```python
from build123d import *

# Parameters (mm, degrees)
SKETCH3_W          = 5
SKETCH3_H          = 2.5
CUT_EXTRUDE1_DEPTH = 14.999635526


with BuildPart() as part:
    # Sketch1 → Revolve1 (revolve)
    with BuildSketch(Plane.XY):
        with BuildLine():
            Line((5, -4.898979486), (5, -9.898979486))
            Line((5, -9.898979486), (0, -9.898979486))
            Line((0, -9.898979486), (0, -5))
            ThreePointArc((0, -5), (4.225771274, -2.672612419), (4.517539515, 2.142857143))
            Line((4.517539515, 2.142857143), (6.32455532, 3))
            ThreePointArc((6.32455532, 3), (6.903611919, -1.157645227), (5, -4.898979486))
        make_face()
    revolve1 = revolve(axis=Axis((0, 12.862963673, 0), (0, -1, 0)))

    # Sketch3 → Cut-Extrude1 (cut, symmetric)
    with BuildSketch(Plane.XY):
        with Locations((0, -8.648979486)):
            Rectangle(SKETCH3_W, SKETCH3_H)
    cut_extrude1 = extrude(amount=CUT_EXTRUDE1_DEPTH, both=True, mode=Mode.SUBTRACT)

    # Mirror1: Revolve1, Cut-Extrude1 across plane
    add(revolve1.mirror(Plane(origin=(5, -9.898979486, 0), x_dir=(0, 0, 1), z_dir=(0, 1, 0))))
    add(cut_extrude1.mirror(Plane(origin=(5, -9.898979486, 0), x_dir=(0, 0, 1), z_dir=(0, 1, 0))), mode=Mode.SUBTRACT)


solid = part.part
```
Source: CAD feature listing. Evaluate the final solid. Frame: model axes, mm. Give positions to 0.01 mm unless a question says otherwise; leave off trailing zeros. Write each loop counter-clockwise with the first axis right and the second up, starting at its lowest first coordinate (ties: lowest second). Pieces come first, ordered by that corner, then holes.
1. Material intervals for line 1 along X through (y, z) = (-11.5, 2.5); line 2 along Y through (x, z) = (4.5, -2.5); line 3 along X through (y, z) = (-3, 1.75), sorted ascending.
2. First-contact query: pin 1 (0.8 mm diameter, centred on y = -8.5, z = 0, fed in from +X); pin 2 (6 mm diameter, centred on y = -13, z = 4.5, fed in from -X); pin 3 (1 mm diameter, centred on x = -1.5, y = 0.5, fed in from +Z). Flat tips, straight axial feed; report the tip coordinate or a pass-through.
3. Section query A-A (z = 0). Return the cut outline in (x, y), then the cut area to 3 significant figures.
4. Section query C-C (y = -11.75). Return the cut outline in (x, z), then the cut area to 3 significant figures.
5. Section query D-D (y = -18.5). Return the cut outline in (x, z).
6. Section query B-B (x = 0). Return the cut outline in (y, z).
Output values:
1. line 1: x = -4.33 to -2.5, 2.5 to 4.33
1. line 2: y = -22.24 to -15.05, -4.74 to 2.44
1. line 3: x = -6.08 to -3.6, 3.6 to 6.08
2. pin 1: stops at x = 5
2. pin 2: stops at x = -4.77
2. pin 3: stops at z = 6.92
3. outline: (-6.32, -22.8) - (-4.52, -21.94) arc R5 cw (long way) to (4.52, -21.94) - (6.32, -22.8) arc R7 ccw to (5, -14.9) - (5, -4.9) arc R7 ccw to (6.32, 3) - (4.52, 2.14) arc R5 cw (long way) to (-4.52, 2.14) - (-6.32, 3) arc R7 ccw to (-5, -4.9) - (-5, -14.9) arc R7 ccw to start; hole (-2.5, -12.4) - (2.5, -12.4) - (2.5, -7.4) - (-2.5, -7.4) - close
3. area: 143 mm2
4. outline: (-2.5, -4.33) - (-2.5, 4.33) arc R5 ccw to start; (2.5, -4.33) arc R5 ccw to (2.5, 4.33) - close
4. area: 30.7 mm2
5. outline: circle Ø13.76 at (0, 0); hole circle Ø9.66 at (0, 0)
6. outline: (-22.8, -6.32) arc R7 ccw to (-14.9, -5) - (-12.4, -5) - (-12.4, 5) - (-14.9, 5) arc R7 ccw to (-22.8, 6.32) - (-21.94, 4.52) arc R5 cw (long way) to (-21.94, -4.52) - close; (-7.4, -5) - (-4.9, -5) arc R7 ccw to (3, -6.32) - (2.14, -4.52) arc R5 cw (long way) to (2.14, 4.52) - (3, 6.32) arc R7 ccw to (-4.9, 5) - (-7.4, 5) - close
